from build123d import *

# Parameters (mm, degrees)
SKETCH_R      = 28.5
PAD_DEPTH     = 2
SKETCH001_R   = 25
SKETCH001_R_2 = 23
PAD001_DEPTH  = 20
CHAMFER_SIZE  = 1.9
FILLET_R      = 1.9


with BuildPart() as part:
    # Sketch → Pad (new body)
    with BuildSketch(Plane.XY):
        Circle(SKETCH_R)
    extrude(amount=PAD_DEPTH)

    # Sketch001 (on Face3 of Pad) → Pad001 (join)
    with BuildSketch(Plane.XY.offset(2)):
        Circle(SKETCH001_R)
        Circle(SKETCH001_R_2, mode=Mode.SUBTRACT)
    extrude(amount=PAD001_DEPTH)

    # Chamfer
    chamfer_edges = [part.edges().sort_by_distance(p)[0] for p in [
        (-25, 0, 22),
    ]]
    chamfer(chamfer_edges, length=CHAMFER_SIZE)

    # Fillet
    fillet_edges = [part.edges().sort_by_distance(p)[0] for p in [
        (-28.5, 0, 0),
    ]]
    fillet(fillet_edges, radius=FILLET_R)


solid = part.part
Source: CAD feature listing. Evaluate the final solid. Frame: model axes, mm. Give positions to 0.01 mm unless a question says otherwise; leave off trailing zeros. Loops run counter-clockwise (first coordinate to the right, second up) from the corner with the lowest first, then second, coordinate; pieces in that order, holes last. Notation, with made-up numbers: (78, 81) -> (93, 81) arc R23 ccw to (93, 89) -> close; hole circle Ø11 at (8, 83.25). An arc over 180 degrees is marked (long way). Use a Markdown table: item, result. Add a question column.
1) Section query A-A, the plane y = 0. Return the cut outline in (x, z).
2) Section query B-B, the plane z = 11.25. Return the cut outline in (x, y), then the cut area to 3 significant figures.
3) Line query: line 1 along Y through (x, z) = (0, 6.5); line 2 along X through (y, z) = (-11, 11.5); line 3 along Z through (x, y) = (-1, 7.5). Output: solid intervals per line, ascending. Write a range as [from, to].
4) First-contact query: pin 1 (4 mm diameter, centred on x = 9, z = 12, fed in from -Y); pin 2 (6 mm diameter, centred on y = -13, z = 9, fed in from +X); pin 3 (5 mm diameter, centred on x = -12.5, z = 13, fed in from +Y); pin 4 (12 mm diameter, centred on x = 17, y = -10, fed in from +Z). Flat tips, straight axial feed; report the tip coordinate or a pass-through.
5) Pull-direction query (Y, two-part tool) for faces 1 (the face through (-0.1, -25.2, 2)), 2 (the face through (-2.994, 22.804, 11.86)), 3 (the face through (23.846, 7.509, 10.923)), 4 (the face through (0, 0, 2)); classes: +Y half, -Y half, draft (parallel to the pull), parting line (faces both ways), or undercut.
Numbers:
| question | item | result |
|---|---|---|
| 1 | outline | (-28.5, 1.9) arc R1.9 ccw to (-26.6, 0) -> (26.6, 0) arc R1.9 ccw to (28.5, 1.9) -> (28.5, 2) -> (25, 2) -> (25, 20.1) -> (23.1, 22) -> (23, 22) -> (23, 2) -> (-23, 2) -> (-23, 22) -> (-23.1, 22) -> (-25, 20.1) -> (-25, 2) -> (-28.5, 2) -> close |
| 2 | outline | circle Ø50 at (0, 0); hole circle Ø46 at (0, 0) |
| 2 | area | 302 mm2 |
| 3 | line 1 | y = [-25, -23], [23, 25] |
| 3 | line 2 | x = [-22.45, -20.2], [20.2, 22.45] |
| 3 | line 3 | z = [0, 2] |
| 4 | pin 1 | stops at y = -24 |
| 4 | pin 2 | stops at x = 22.91 |
| 4 | pin 3 | stops at y = 22.91 |
| 4 | pin 4 | stops at z = 22 |
| 5 | face 1 | draft |
| 5 | face 2 | undercut |
| 5 | face 3 | parting line |
| 5 | face 4 | undercut |
